Verification items for the finished model (mm, model axes). A direction names the side the tool comes from. Round coordinates to 2 decimals unless told otherwise and drop trailing zeros. Write each loop counter-clockwise with the first axis right and the second up, starting at its lowest first coordinate (ties: lowest second). Pieces come first, ordered by that corner, then holes. Notation, with made-up numbers: (-24.5, 78) - (-4.5, 78) arc R31 cw to (-4.5, 103) - close; hole circle Ø7 at (-28, 22.25). An arc over 180 degrees is marked (long way). Answer as a JSON object with one key per item and string values. Group by question number.
1) Section check D-D (y = 3.25). Enter the section's corners in (x, z).
2) Thickness scan on line 1 (Y direction, x = 2.5, z = 12.5); line 2 (X direction, y = -0.35, z = 19); line 3 (Z direction, x = 11.25, y = 10.5). Record the ranges inside material, lowest first.
3) Set-up check for faces 4 (the cylindrical face through (5.72, 5.3, -1.23)), 5 (the flat face through (0, 4, -0.737)), 6 (the cylindrical face through (5.703, 14.772, -1.23)), 7 (the flat face through (0, 15, 0)), 8 (the cylindrical face through (0.45, -0.49, 10)): record each of +Z, -Z, +X, -X, +Y, -Y from which the full face is reachable in a straight line by a thin tool's end or side.
4) Section check A-A (y = 10.5). Enter the section's corners in (x, z).
5) Section check B-B (z = 21). Enter the section's corners in (x, y), then the cut area to 3 significant figures.
6) Mould release check, pull along Y, two halves, no side actions. Record for faces 1 (the cylindrical face through (0.196, -0.505, -1.214)), 2 (the flat face through (6.004, 10, -1)), 3 (the flat face through (0, 3, -1.737)): +Y half, -Y half, draft (parallel to the pull), parting line (faces both ways), or undercut.
7) Section check C-C (x = 10.75). Enter the section's corners in (y, z), then the cut area to 3 significant figures.
8) Go/stop test with flat-tipped pins: pin 1 Ø0.5 at (y, z) = (-0.5, 13) entering from +X; pin 2 Ø8 at (x, z) = (1.5, 17.5) entering from +Y; pin 3 Ø1.5 at (x, y) = (11, 3) entering from +Z; pin 4 Ø6.5 at (x, z) = (0.41, 19) entering from -Y. Record where each tip stops, or that it passes through.
```python
from build123d import *

# Parameters (mm, degrees)
BASE_FLANGE1_DEPTH = 1
EDGE_FLANGE1_DEPTH = 28
HEM1_START         = -14
HEM1_DEPTH         = 28
HEM1_2_DEPTH       = 28
CUT_EXTRUDE1_DEPTH = 10
CUT_EXTRUDE3_DEPTH = 10


# Read off the part's stored shape, not the designer's step: Hem1
# Sheet-metal steps are written as plain solids
with BuildPart() as part:
    # Sketch1 → Base-Flange1 (new body)
    with BuildSketch(Plane(origin=(0, 0, 0), x_dir=(1, 0, 0), z_dir=(0, 1, 0))):
        with BuildLine():
            Line((-14, 0), (14, 0))
            Line((14, 0), (14, -9))
            Line((14, -9), (7.635806501, -22.426557457))
            ThreePointArc((7.635806501, -22.426557457), (0.597605148, -26.997723985), (-6.650589662, -22.767415048))
            Line((-6.650589662, -22.767415048), (-14, -9))
            Line((-14, -9), (-14, 0))
        make_face()
    extrude(amount=-BASE_FLANGE1_DEPTH)

    # Edge-Flange1 section (across the edge) → Edge-Flange1 (add)
    with BuildSketch(Plane(origin=(14, 0, -0.7366), x_dir=(0, 0, 1), z_dir=(-1, 0, 0))):
        with BuildLine():
            Line((-1, 0.7366), (-1, 19))
            Line((-1, 19), (0, 19))
            Line((0, 19), (0, 0.7366))
            ThreePointArc((0, 0.7366), (0.215745145, 0.215745145), (0.7366, 0))
            Line((0.7366, 0), (0.7366, -1))
            ThreePointArc((0.7366, -1), (-0.491361636, -0.491361636), (-1, 0.7366))
        make_face()
    extrude(amount=EDGE_FLANGE1_DEPTH)

    # Hem1 outline → Hem1 (cut)
    with BuildSketch(Plane.YZ.offset(HEM1_START)):
        with BuildLine():
            Line((19, -0.7366), (18.998808848, -0.7366))
            ThreePointArc((18.998808848, -0.7366), (18.674568837, -1.446534208), (17.95, -1.7366))
            Line((17.95, -1.7366), (19, -1.7366))
            Line((19, -1.7366), (19, -0.7366))
        make_face()
    extrude(amount=HEM1_DEPTH, mode=Mode.SUBTRACT)

    # Hem1 2 outline → Hem1 2 (add)
    with BuildSketch(Plane.YZ.offset(HEM1_START)):
        with BuildLine():
            Line((15, 0.3634), (15, -0.6366))
            Line((15, -0.6366), (17.95, -0.6366))
            ThreePointArc((17.95, -0.6366), (18, -0.6866), (17.95, -0.7366))
            Line((17.95, -0.7366), (18.998808848, -0.7366))
            ThreePointArc((18.998808848, -0.7366), (18.709934208, 0.037968837), (17.95, 0.3634))
            Line((17.95, 0.3634), (15, 0.3634))
        make_face()
    extrude(amount=HEM1_2_DEPTH)

    # Sketch15 → Cut-Extrude1 (cut)
    with BuildSketch(Plane.XY.offset(-0.7366)):
        with BuildLine():
            Line((-5.004090335, 15.057117645), (5.004090335, 15.057117645))
            ThreePointArc((5.004090335, 15.057117645), (5.711197117, 14.764224427), (6.004090335, 14.057117645))
            Line((6.004090335, 14.057117645), (6.004090335, 6))
            ThreePointArc((6.004090335, 6), (5.711197117, 5.292893219), (5.004090335, 5))
            Line((5.004090335, 5), (-5.004090335, 5))
            ThreePointArc((-5.004090335, 5), (-5.711197117, 5.292893219), (-6.004090335, 6))
            Line((-6.004090335, 6), (-6.004090335, 14.057117645))
            ThreePointArc((-6.004090335, 14.057117645), (-5.711197117, 14.764224427), (-5.004090335, 15.057117645))
        make_face()
    extrude(amount=-CUT_EXTRUDE1_DEPTH, mode=Mode.SUBTRACT)

    # Sketch16 → Cut-Extrude3 (cut)
    with BuildSketch(Plane(origin=(0, 0, 0), x_dir=(1, 0, 0), z_dir=(0, 1, 0))):
        with BuildLine():
            Line((-1.593211689, -12), (-1.593211689, -14.527864045))
            ThreePointArc((-1.593211689, -14.527864045), (-1.767469831, -15.344360626), (-2.259878356, -16.01857603))
            ThreePointArc((-2.259878356, -16.01857603), (0.406788311, -23), (3.073454977, -16.01857603))
            ThreePointArc((3.073454977, -16.01857603), (2.581046452, -15.344360626), (2.406788311, -14.527864045))
            Line((2.406788311, -14.527864045), (2.406788311, -12))
            ThreePointArc((2.406788311, -12), (0.406788311, -10), (-1.593211689, -12))
        make_face()
    extrude(amount=-CUT_EXTRUDE3_DEPTH, mode=Mode.SUBTRACT)


solid = part.part
```
Returned:
{
 "1": {"outline": "(-14, -1.74) - (14, -1.74) - (14, -0.74) - (-14, -0.74) - close"},
 "2": {"line 1": "-1 to 0", "line 2": "-8.66 to -3.59, 4.41 to 9.26", "line 3": "-1.74 to -0.74"},
 "3": {"face 4": "+Z, -Z", "face 5": "+X, -X", "face 6": "-Z", "face 7": "+Z, +X, -X", "face 8": "+Y, -Y"},
 "4": {"outline": "(-14, -1.74) - (-6, -1.74) - (-6, -0.74) - (-14, -0.74) - close; (6, -1.74) - (14, -1.74) - (14, -0.74) - (6, -0.74) - close"},
 "5": {"outline": "(-7.59, -1) - (-3.06, -1) - (-3.06, 0) - (-7.59, 0) - close; (3.87, -1) - (8.31, -1) - (8.31, 0) - (3.87, 0) - close", "area": "8.98 mm2"},
 "6": {"face 1": "-Y half", "face 2": "undercut", "face 3": "draft"},
 "7": {"outline": "(-1, 0) arc R1.74 ccw to (0.74, -1.74) - (17.95, -1.74) arc R1.05 ccw to (17.95, 0.36) - (15, 0.36) - (15, -0.64) - (17.95, -0.64) arc R0.05 cw to (17.95, -0.74) - (0.74, -0.74) arc R0.74 cw to (0, 0) - (0, 15.86) - (-1, 15.86) - close", "area": "39.7 mm2"},
 "8": {"pin 1": "x = 12.22", "pin 2": "y = 0", "pin 3": "z = -0.74", "pin 4": "through"}
}
